Read the model definition and answer for the solid it produces. Units are mm, in the model's axes. A direction names the side the tool comes from. Coordinates: 2 decimals unless noted, no trailing zeros. Write each loop counter-clockwise with the first axis right and the second up, starting at its lowest first coordinate (ties: lowest second). Pieces come first, ordered by that corner, then holes.
(1) Which of the six approach directions +Z, -Z, +X, -X, +Y, -Y give full straight-line access (tool end or side, diameter ignored) to faces 1 (the flat face through (25, 0, 0)), 2 (the cylindrical face through (12.43, -0.54, -2.44))?
(2) Given pin 1 (2 mm diameter, centred on x = 16.5, z = 2, fed in from -Y); pin 2 (4 mm diameter, centred on x = 10, y = 0.5, fed in from +Z); pin 3 (3 mm diameter, centred on x = 10.5, z = -3, fed in from +Y), each flat-ended and moving along its own axis, determine where each tip first touches the part or whether it passes through.
(3) Section A-A on x = 8.5 is taken. Write down the section's boundary in (y, z).
(4) Find the intervals of material crossed by probe 1 along Z at (x, y) = (23.25, 1.5); probe 2 along X at (y, z) = (2.75, -2.5); probe 3 along X at (y, z) = (2.5, 2), in increasing order.
Autodesk Inventor part; units mm, degrees
ref_plane "Work Plane1" through (1.525, 0, 0) normal (0, 0, 1) x (1, 0, 0)
ref_plane "YZ Plane" through (0, 0, 0) normal (1, 0, 0) x (0, 1, 0)
ref_plane "XZ Plane" through (0, 0, 0) normal (0, 1, 0) x (-1, 0, 0)
sketch "Szkic1" plane through (0, 0, 0) normal (0, 0, 1) x (1, 0, 0)
  line L0 (0, 3.6) -> (0, 2.5)
  line L1 (9, 2.5) -> (25, 2.5)
  line L2 (25, 2.5) -> (25, 0)
  line L3 (25, 0) -> (-0.2001, 0)
  line L4 (-5.2401, 0) -> (30.04, 0)
  line L5 (-0.2001, 0) -> (-0.2001, 3.6)
  line L6 (-0.2001, 3.6) -> (0, 3.6)
  line L7 (9, 2.5) -> (8.5091, 2.5)
  line L8 (8.5091, 2.5) -> (0, 2.5)
  line L9 (0, -0.72) -> (0, 4.32)
  dimension "d0" = 25
  dimension "d1" = 16
  dimension "d2" = 5
  dimension "d9" = 0.2001
  dimension "d10" = 7.2
  dimension "d13" = 0.4909
  dimension "d14" = 5
revolve "Bryła" add sketch "Szkic1" angle 360 about axis through (25, 0, 0) along (-1, 0, 0)
sketch "Szkic2" plane through (-0.2001, 0, 0) normal (-1, 0, 0) x (0, 0, 1)
  line L0 (0, 4.6188) -> (4, 2.3094)
  line L1 (4, 2.3094) -> (4, -2.3094)
  line L2 (4, -2.3094) -> (0, -4.6188)
  line L3 (0, -4.6188) -> (-4, -2.3094)
  line L4 (-4, -2.3094) -> (-4, 2.3094)
  line L5 (-4, 2.3094) -> (0, 4.6188)
  point P0 (0, 0)
  point P1 (0, 0)
  dimension "d11" = 8
extrude "Głowica" add sketch "Szkic2" along normal blind 3.45
sketch "Szkic4" plane through (0, 0, 0) normal (0, 0, 1) x (1, 0, 0)
  line L0 (-3.6501, 4) -> (-3.6501, 4.6188)
  line L1 (-3.6501, 4.6188) -> (-3.2928, 4.6188)
  line L2 (-3.2928, 4.6188) -> (-3.6501, 4)
  line L3 (-4.3401, 0) -> (0.4899, 0)
  line L4 (-0.2001, 4.6188) -> (-3.6501, 4.6188)
  line L5 (-3.6501, 2.3094) -> (-3.6501, 4.6188)
  dimension "d5" = 30
  dimension "d19" = 8
revolve "Faza1" cut sketch "Szkic4" angle 360 about axis through (-10, 0, 0) along (1, 0, 0)
thread "Gwint"
chamfer "Faza2" distance 0.4908 distance2 0.4909 1 edges at (25, -2.5, 0) measured on face at (25, 0.7379, -0.3873)
ref_plane "Work Plane1" through (1.525, 0, 0) normal (0, 0, 1) x (1, 0, 0)
equation "\"d0\" = NLG"
equation "\"d1\" = GEL"
equation "\"d2\" = GD"
equation "\"d10\" = SD2"
equation "\"d14\" = BDM"
equation "\"d11\" = SW"
equation "\"d3\" = KOH - SD"
equation "\"d5\" = ANG1"
equation "\"d19\" = SW0"
equation "\"d15\" = GEL"
equation "\"d6\" = -0.5 * SPD + 0.5 * GD"
equation "\"NLG\" = 25"
equation "\"GD\" = NND"
equation "\"BDM\" = NND"
equation "\"KOH\" = 3.65"
equation "\"GEL\" = 16"
equation "\"SW\" = 8"
equation "\"SW0\" = 8"
equation "\"SPD\" = NND - 1.2269 * PTC"
equation "\"SD2\" = 0.9 * SW"
equation "\"SD\" = 0.2"
equation "\"ANG1\" = 30deg"
equation "\"GAL\" = 0.61345 * PTC"
equation "\"GUL\" = 0.61345 * PTC"
equation "\"RR\" = 0.35"
equation "\"GD1\" = THREADDIA - 1.2269 * PTC"
equation "\"THREADDIA\" = 5"
equation "\"SDH\" = 7.55"
equation "\"TOA\" = 30deg"
equation "\"PTC\" = 0.8"
equation "\"NND\" = 5"
equation "\"E0\" = 1.155 * SW"
properties part number "BS 3692 - M5 x 25" material "Stal, miękka"
Response:
1. face 1: +Z, -Z, +X, +Y, -Y
1. face 2: +X
2. pin 1: stops at y = -2.29
2. pin 2: stops at z = 2.5
2. pin 3: stops at y = 2
3. outline: circle Ø5 at (0, 0)
4. probe 1: z = -2 to 2
4. probe 2: x = -3.65 to -0.2
4. probe 3: x = -3.65 to 0
